For this review, take the finished solid that the model builds, in its own axes (mm). A direction names the side the tool comes from. Coordinates: 2 decimals unless noted, no trailing zeros. Loops run counter-clockwise (first coordinate to the right, second up) from the corner with the lowest first, then second, coordinate; pieces in that order, holes last. Notation, with made-up numbers: (-3.75, 25.5) -> (35.25, 25.5) arc R16 ccw to (35.25, 45.5) -> close; hole circle Ø5 at (36, -28.5). An arc over 180 degrees is marked (long way). Use a Markdown table: item, result.
from build123d import *

# Parameters (mm, degrees)
F1_DEPTH      = 7.5
F2_W          = 5
F2_H          = 3.6
F3_DEPTH      = 5
F3_DEPTH_BACK = 12.5
F5_DEPTH      = 35.2
F6_R          = 1.5
F6_R_2        = 1.25
F7_DEPTH      = 25


with BuildPart() as f1:
    # F0 (on Front) → F1 (new body)
    with BuildSketch(Plane.XZ):
        with BuildLine():
            Line((16.9, 3.6), (11.9, 3.6))
            ThreePointArc((11.9, 3.6), (9.3, 1), (6.7, 3.6))
            Line((6.7, 3.6), (5.7, 3.6))
            ThreePointArc((5.7, 3.6), (3.1, 1), (0.5, 3.6))
            Line((0.5, 3.6), (-0.5, 3.6))
            ThreePointArc((-0.5, 3.6), (-3.1, 1), (-5.7, 3.6))
            Line((-5.7, 3.6), (-6.7, 3.6))
            ThreePointArc((-6.7, 3.6), (-9.3, 1), (-11.9, 3.6))
            Line((-11.9, 3.6), (-16.9, 3.6))
            Line((-16.9, 3.6), (-16.9, 0))
            Line((-16.9, 0), (16.9, 0))
            Line((16.9, 0), (16.9, 3.6))
        make_face()
    extrude(amount=F1_DEPTH)

    # F2 (on face) → F3 (join, two sides)
    with BuildSketch(Plane(origin=(0, 0, 0), x_dir=(-1, 0, 0), z_dir=(0, 1, 0))) as f3_sk:
        with Locations((-14.4, 1.8)):
            Rectangle(F2_W, F2_H)
        with Locations((14.4, 1.8)):
            Rectangle(F2_W, F2_H)
    extrude(amount=F3_DEPTH)
    extrude(f3_sk.sketch, amount=-F3_DEPTH_BACK)

    # F4 (on face) → F5 (cut)
    with BuildSketch(Plane.YZ.offset(16.9)):
        Polygon((-7.5, 3.6), (-12.5, 3.6), (-12.5, 0), align=None)
        Polygon((5, 0), (5, 3.6), (0, 3.6), align=None)
    extrude(amount=-F5_DEPTH, mode=Mode.SUBTRACT)

    # F6 (on face) → F7 (cut)
    with BuildSketch(Plane(origin=(0, 0, 0), x_dir=(1, 0, 0), z_dir=(0, 0, -1))):
        with Locations((14.4, 10)):
            Circle(F6_R)
        with Locations((14.4, 3.75)):
            Circle(F6_R_2)
        with Locations((14.4, -2.5)):
            Circle(F6_R)
        with Locations((-14.4, -2.5)):
            Circle(F6_R)
        with Locations((-14.4, 10)):
            Circle(F6_R)
        with Locations((-14.4, 3.75)):
            Circle(F6_R_2)
    extrude(amount=-F7_DEPTH, mode=Mode.SUBTRACT)


solid = f1.part
(1) For line 1 along X through (y, z) = (-10, 1.25); line 2 along Y through (x, z) = (-14.4, 0.6); line 3 along Y through (x, z) = (7, 1.05), list the stretches that pass through material, from the lowest coordinate up.
Found:
| item | result |
|---|---|
| line 1 | x = -16.9 to -15.9, -12.9 to -11.9, 11.9 to 12.9, 15.9 to 16.9 |
| line 2 | y = -11.67 to -11.5, -8.5 to -5, -2.5 to 1, 4 to 4.17 |
| line 3 | y = -7.5 to 0 |
(2) For pin 1 Ø1.8 at (y, z) = (3.5, 1.5) entering from +X; pin 2 Ø1.5 at (x, y) = (-14.4, -3.75) entering from -Z; pin 3 Ø1.5 at (x, y) = (-13, 1) entering from +Z; pin 4 Ø3.5 at (x, y) = (-14.4, 2.5) entering from +Z, all flat-tipped, find the tip position at first contact; note any pin that passes through.
Found:
| item | result |
|---|---|
| pin 1 | stops at x = 16.9 |
| pin 2 | passes through |
| pin 3 | stops at z = 3.42 |
| pin 4 | stops at z = 3.06 |
(3) Mouldability with a two-part tool opening along X and no side actions: class faces 1 (the face through (-11.9, 2, 1)), 2 (the face through (-3, -4, 1)), 3 (the face through (16.9, -4, 1)), 4 (the face through (0, -4, 0)) as pulls with the +X half, pulls with the -X half, needs draft (parallel to the pull), parting line crosses it, or undercut.
Found:
| item | result |
|---|---|
| face 1 | undercut |
| face 2 | undercut |
| face 3 | pulls with the +X half |
| face 4 | needs draft |
(4) For faces 5 (the face through (0, -7.5, 1)), 6 (the face through (0, 0, 1)), 7 (the face through (14.205, 1.013, 1.1)), list the 3-axis set-ups (+Z, -Z, +X, -X, +Y, -Y) from which the entire face can be reached by the end or side of a thin tool; tool diameter is ignored.
Found:
| item | result |
|---|---|
| face 5 | +Z, -Z, -Y |
| face 6 | +Z, -Z, +Y |
| face 7 | +Z, -Z |
(5) Take a section at D-D on y = -6.5. Write out the cut boundary in (x, z).
Found:
| item | result |
|---|---|
| outline | (-16.9, 0) -> (16.9, 0) -> (16.9, 3.6) -> (11.9, 3.6) arc R2.6 cw to (6.7, 3.6) -> (5.7, 3.6) arc R2.6 cw to (0.5, 3.6) -> (-0.5, 3.6) arc R2.6 cw to (-5.7, 3.6) -> (-6.7, 3.6) arc R2.6 cw to (-11.9, 3.6) -> (-16.9, 3.6) -> close |
(6) Take a section at B-B on z = 3.25. State how many separate pieces and enclosed holes the cut face has, plus the area to 3 significant figures.
Found:
| item | result |
|---|---|
| separate pieces | 5 |
| enclosed holes | 2 |
| area | 98.8 mm^2 |
(7) Take a section at C-C on y = 2.5. Write out the cut boundary in (x, z), plus the area to 3 significant figures.
Found:
| item | result |
|---|---|
| outline | (-16.9, 0) -> (-15.9, 0) -> (-15.9, 1.8) -> (-16.9, 1.8) -> close; (-12.9, 0) -> (-11.9, 0) -> (-11.9, 1.8) -> (-12.9, 1.8) -> close; (11.9, 0) -> (12.9, 0) -> (12.9, 1.8) -> (11.9, 1.8) -> close; (15.9, 0) -> (16.9, 0) -> (16.9, 1.8) -> (15.9, 1.8) -> close |
| area | 7.20 mm^2 |
(8) Take a section at A-A on x = 14.4. Write out the cut boundary in (y, z), plus the area to 3 significant figures.
Found:
| item | result |
|---|---|
| outline | (-12.5, 0) -> (-11.5, 0) -> (-11.5, 0.72) -> close; (-8.5, 0) -> (-5, 0) -> (-5, 3.6) -> (-7.5, 3.6) -> (-8.5, 2.88) -> close; (-2.5, 0) -> (1, 0) -> (1, 2.88) -> (0, 3.6) -> (-2.5, 3.6) -> close; (4, 0) -> (5, 0) -> (4, 0.72) -> close |
| area | 25.2 mm^2 |
